Build history of the part. All positions in model axes, mm. A direction names the side the tool comes from. Round coordinates to 2 decimals unless told otherwise and drop trailing zeros. Write each loop counter-clockwise with the first axis right and the second up, starting at its lowest first coordinate (ties: lowest second). Pieces come first, ordered by that corner, then holes. Notation, with made-up numbers: (49.5, -37.5) -> (106.5, -37.5) arc R14 cw to (106.5, -25.5) -> close; hole circle Ø5 at (-35, 44). An arc over 180 degrees is marked (long way). One line per question, with ' | ' between items.
from build123d import *

# Parameters (mm, degrees)
BOSS_EXTRUDE1_DEPTH = 7.9375
SKETCH3_R           = 5.207
CUT_EXTRUDE1_DEPTH  = 3.96875
SKETCH4_R           = 1.2065
BOSS_EXTRUDE2_DEPTH = 12.065


with BuildPart() as part:
    # Sketch1 → Boss-Extrude1 (new, symmetric)
    with BuildSketch(Plane(origin=(0, 0, 0), x_dir=(1, 0, 0), z_dir=(0, 1, 0))):
        Polygon((-2.757708096, -19.86108723), (1.211041904, -19.86108723), (1.211041904, 41.25766277), (58.361041904, 41.25766277), (58.361041904, 45.22641277), (6.27967861, 45.22641277), (-2.757708096, 45.22641277), align=None)
    extrude(amount=BOSS_EXTRUDE1_DEPTH, both=True)

    # Sketch3 → Cut-Extrude1 (cut)
    with BuildSketch(Plane.ZY.offset(2.757708096)):
        with Locations((-12.566559842, 0)):
            Circle(SKETCH3_R)
    extrude(amount=-CUT_EXTRUDE1_DEPTH, mode=Mode.SUBTRACT)

    # Sketch4 → Boss-Extrude2 (add)
    with BuildSketch(Plane(origin=(0, 0, -45.22641277), x_dir=(-1, 0, 0), z_dir=(0, 0, -1))):
        with Locations(Location((-37.564791904, 0, 0), (0, 0, 180))):
            Circle(SKETCH4_R)
    extrude(amount=BOSS_EXTRUDE2_DEPTH)


solid = part.part
(1) Slice it at C-C (y = 4). Write the cut outline in (x, z), then the cut area to 3 significant figures.
Calculated:
outline: (-2.76, -45.23) -> (58.36, -45.23) -> (58.36, -41.26) -> (1.21, -41.26) -> (1.21, -15.9) -> (-2.76, -15.9) -> close; (-2.76, -9.23) -> (1.21, -9.23) -> (1.21, 19.86) -> (-2.76, 19.86) -> close | area: 459 mm2
(2) 3-axis set-ups, long thin cutter, end or side, ignore diameter. For faces 4 (the flat face through (-1, 0, 19.861)), 5 (the cylindrical face through (38.716, -0.362, -51.174)): which of +Z, -Z, +X, -X, +Y, -Y reach the whole face in a straight line?
Calculated:
face 4: +Z, +X, -X, +Y, -Y | face 5: -Z
(3) Drop flat-ended pins along their axis: pin 1 (8 mm diameter, centred on x = 24, y = -2.5, fed in from -Z); pin 2 (9.5 mm diameter, centred on y = 0, z = -12.57, fed in from +X); pin 3 (6 mm diameter, centred on y = -4, z = -19.5, fed in from +X); pin 4 (1 mm diameter, centred on x = 52, y = 0, fed in from +Z). Give the stop position or say it passes through.
Calculated:
pin 1: z = -45.23 | pin 2: through | pin 3: x = 1.21 | pin 4: z = -41.26
(4) Wall check: line 1 (X direction, y = -4, z = 8.5); line 2 (Z direction, x = 31.5, y = 6); line 3 (Y direction, x = 0, z = -14.5). Give the ranges that are in metal, low to high. Write a range as from..to.
Calculated:
line 1: -2.76..1.21 | line 2: -45.23..-41.26 | line 3: -7.94..-4.83, 4.83..7.94
(5) Mould opens along Z. For faces 1 (the cylindrical face through (-0.8, 1.56, -7.6)), 2 (the flat face through (29, 0, -41.258)), 3 (the flat face through (1.211, -5, -10)) say: pulls with the +Z half, pulls with the -Z half, needs draft (parallel to the pull), parting line crosses it, or undercut.
Calculated:
face 1: undercut | face 2: pulls with the +Z half | face 3: needs draft
(6) Slice it at B-B (z = -50). Write the cut outline in (x, y), then the cut area to 3 significant figures.
Calculated:
outline: circle Ø2.41 at (37.56, 0) | area: 4.57 mm2
(7) Slice it at D-D (x = 49.5). Write the cut outline in (y, z).
Calculated:
outline: (-7.94, -45.23) -> (7.94, -45.23) -> (7.94, -41.26) -> (-7.94, -41.26) -> close
(8) Slice it at A-A (y = 0). Write the cut outline in (x, z), then the cut area to 3 significant figures.
Calculated:
outline: (-2.76, -45.23) -> (36.36, -45.23) -> (36.36, -57.29) -> (38.77, -57.29) -> (38.77, -45.23) -> (58.36, -45.23) -> (58.36, -41.26) -> (1.21, -41.26) -> (1.21, -17.77) -> (-2.76, -17.77) -> close; (-2.76, -7.36) -> (1.21, -7.36) -> (1.21, 19.86) -> (-2.76, 19.86) -> close | area: 473 mm2
